Drawing for the job (mm, zero at the part's lowest x, y, z). A direction names the side the tool comes from. Round coordinates to 2 decimals unless told otherwise and drop trailing zeros. Write each loop counter-clockwise with the first axis right and the second up, starting at its lowest first coordinate (ties: lowest second). Pieces come first, ordered by that corner, then holes. Notation, with made-up numbers: (46.25, 62.5) -> (100.25, 62.5) arc R10 ccw to (100.25, 74.5) -> close; hole circle Ø7 at (45.5, 70.25). An arc over 180 degrees is marked (long way). One line per question, with ' | ' between items.
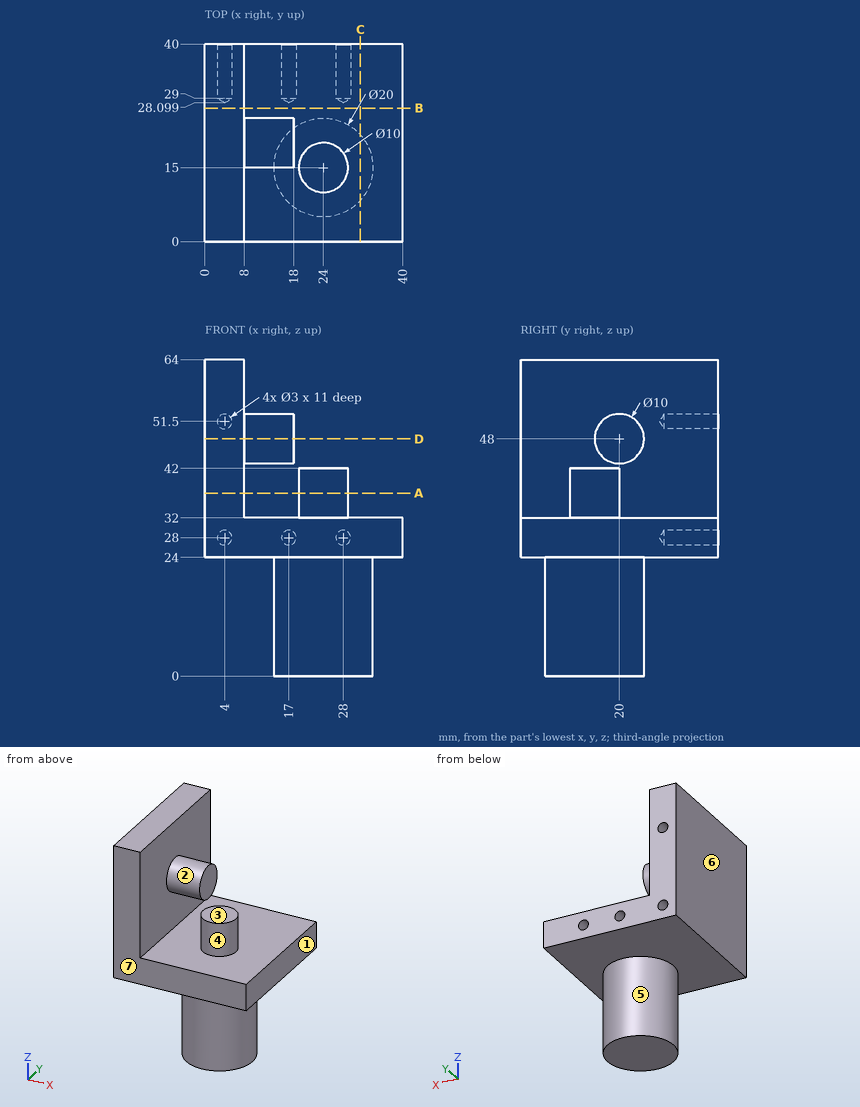
(1) Wall check: line 1 (X direction, y = 32, z = 28); line 2 (Z direction, x = 4, y = 37.25); line 3 (Z direction, x = 17, y = 36.75). Give the ranges that are in metal, low to high. Write a range as from..to.
Calculated:
line 1: 0..2.5, 5.5..15.5, 18.5..26.5, 29.5..40 | line 2: 24..26.5, 29.5..50, 53..64 | line 3: 24..26.5, 29.5..32
(2) Slice it at C-C (x = 31.5). Write the cut outline in (y, z).
Calculated:
outline: (0, 24) -> (8.39, 24) -> (8.39, 0) -> (21.61, 0) -> (21.61, 24) -> (40, 24) -> (40, 32) -> (0, 32) -> close
(3) Slice it at B-B (y = 27). Write the cut outline in (x, z).
Calculated:
outline: (0, 24) -> (40, 24) -> (40, 32) -> (8, 32) -> (8, 64) -> (0, 64) -> close
(4) 3-axis set-ups, long thin cutter, end or side, ignore diameter. For the marked faces 1, 2 and 3: which of +Z, -Z, +X, -X, +Y, -Y reach the whole face in a straight line?
Calculated:
face 1: +Z, -Z, +X, +Y, -Y | face 2: +X | face 3: +Z, +X, +Y, -Y
(5) Drop flat-ended pins along their axis: pin 1 (3 mm diameter, centred on y = 19.5, z = 48, fed in from +X); pin 2 (8 mm diameter, centred on x = 34.5, y = 34.5, fed in from -Z); pin 3 (2.5 mm diameter, centred on x = 4, z = 28, fed in from +Y). Give the stop position or say it passes through.
Calculated:
pin 1: x = 18 | pin 2: z = 24 | pin 3: y = 28.85
(6) Slice it at D-D (z = 48). Write the cut outline in (x, y).
Calculated:
outline: (0, 0) -> (8, 0) -> (8, 15) -> (18, 15) -> (18, 25) -> (8, 25) -> (8, 40) -> (0, 40) -> close
(7) Slice it at A-A (z = 37). Write the cut outline in (x, y).
Calculated:
outline: (0, 0) -> (8, 0) -> (8, 40) -> (0, 40) -> close; circle Ø10 at (24, 15)
(8) Mould opens along X. For the marked faces 4, 5, 6 and 7 say: pulls with the +X half, pulls with the -X half, needs draft (parallel to the pull), parting line crosses it, or undercut.
Calculated:
face 4: undercut | face 5: parting line crosses it | face 6: pulls with the -X half | face 7: needs draft
